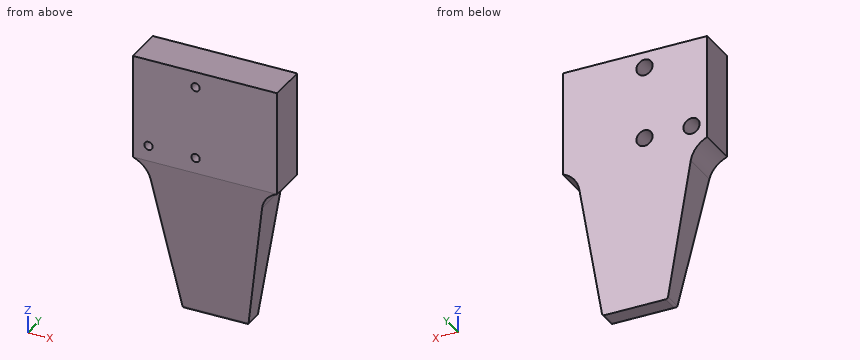
from build123d import *

# Parameters (mm, degrees)
SKETCH1_W           = 55.25
SKETCH1_H           = 100
SKETCH1_R           = 1.6
BOSS_EXTRUDE1_DEPTH = 15
SKETCH2_R           = 3.1
CUT_EXTRUDE1_DEPTH  = 7.5
CUT_EXTRUDE3_REACH  = 117.228
CUT_EXTRUDE2_REACH  = 117.228
FILLET3_R           = 10
FILLET4_R           = 1


with BuildPart() as part:
    # Sketch1 → Boss-Extrude1 (new body)
    with BuildSketch(Plane(origin=(0, 0, 0), x_dir=(1, 0, 0), z_dir=(0, 1, 0))):
        with Locations((27.625, 50)):
            Rectangle(SKETCH1_W, SKETCH1_H)
        with Locations(Location((24, 6, 0), (0, 0, 270))):
            Circle(SKETCH1_R, mode=Mode.SUBTRACT)
        with Locations(Location((6, 34, 0), (0, 0, 270))):
            Circle(SKETCH1_R, mode=Mode.SUBTRACT)
        with Locations(Location((24, 34, 0), (0, 0, 270))):
            Circle(SKETCH1_R, mode=Mode.SUBTRACT)
    extrude(amount=BOSS_EXTRUDE1_DEPTH)

    # Sketch2 → Cut-Extrude1 (cut)
    with BuildSketch(Plane(origin=(0, 15, 0), x_dir=(1, 0, 0), z_dir=(0, 1, 0))):
        with Locations(Location((24, 34, 0), (0, 0, 270))):
            Circle(SKETCH2_R)
        with Locations(Location((24, 6, 0), (0, 0, 270))):
            Circle(SKETCH2_R)
        with Locations(Location((6, 34, 0), (0, 0, 270))):
            Circle(SKETCH2_R)
    extrude(amount=-CUT_EXTRUDE1_DEPTH, mode=Mode.SUBTRACT)

    # Sketch5 → Cut-Extrude3 (cut, up to next)
    with BuildSketch(Plane(origin=(55.25, 0, 0), x_dir=(0, 0, -1), z_dir=(1, 0, 0)), mode=Mode.PRIVATE) as cut_extrude3_sk1:
        Polygon((40, 0), (100, 8), (100, 0), align=None)
    cut_extrude3_tool1 = extrude(cut_extrude3_sk1.sketch, amount=-CUT_EXTRUDE3_REACH, mode=Mode.PRIVATE) & part.part
    add(cut_extrude3_tool1.solids().sort_by_distance((55.25, 2.666667, -80))[0], mode=Mode.SUBTRACT)

    # Sketch3 → Cut-Extrude2 (cut, up to next)
    with BuildSketch(Plane(origin=(0, 15, 0), x_dir=(1, 0, 0), z_dir=(0, 1, 0)), mode=Mode.PRIVATE) as cut_extrude2_sk1:
        Polygon((40.125, 100), (55.25, 100), (55.25, 40), (50.25, 40), align=None)
    cut_extrude2_tool1 = extrude(cut_extrude2_sk1.sketch, amount=-CUT_EXTRUDE2_REACH, mode=Mode.PRIVATE) & part.part
    # Sketch3 → Cut-Extrude2 (cut, up to next)
    with BuildSketch(Plane(origin=(0, 15, 0), x_dir=(1, 0, 0), z_dir=(0, 1, 0)), mode=Mode.PRIVATE) as cut_extrude2_sk2:
        Polygon((15.125, 100), (0, 100), (0, 40), (5, 40), align=None)
    cut_extrude2_tool2 = extrude(cut_extrude2_sk2.sketch, amount=-CUT_EXTRUDE2_REACH, mode=Mode.PRIVATE) & part.part
    add(cut_extrude2_tool1.solids().sort_by_distance((49.794255, 15, -75.031056))[0], mode=Mode.SUBTRACT)
    add(cut_extrude2_tool2.solids().sort_by_distance((5.455745, 15, -75.031056))[0], mode=Mode.SUBTRACT)

    # Fillet3
    # the kernel refuses this fillet: 10 mm, written as the material it adds along each edge
    with BuildSketch(Plane(origin=(5, 15, -40), x_dir=(-1, 0, 0), z_dir=(0, -1, 0))) as fillet3_piece_1_section:
        with BuildLine():
            CenterArc((8.564743476, 9.343051105), FILLET3_R, 189.578422919, 59.537746257)
            Line((-1.295844232, 7.679076929), (-1.493055986, 7.645797446))
            Line((-1.493055986, 7.645797446), (-0.197211754, -0.033279484))
            Line((-0.197211754, -0.033279484), (0, -0.2))
            ThreePointArc((0, -0.2), (2.5, -0.2), (4.92870513, -0.186861022))
            Line((4.92870513, -0.186861022), (5, 0))
        make_face()
    fillet3_piece_1 = extrude(amount=15, mode=Mode.PRIVATE)
    fillet3_piece_1 = split(fillet3_piece_1, bisect_by=Plane(origin=(4.040002964, 0.373004519, -42.797533893), z_dir=(0, 0.9912279006826347, 0.13216372009101796)), keep=Keep.TOP, mode=Mode.PRIVATE)
    add(fillet3_piece_1)
    with BuildSketch(Plane(origin=(50.25, 15, -40), x_dir=(1, 0, 0), z_dir=(0, -1, 0))) as fillet3_piece_2_section:
        with BuildLine():
            CenterArc((8.564743476, -9.343051105), FILLET3_R, 110.883830823, 59.537746257)
            Line((-1.295844232, -7.679076929), (-1.493055986, -7.645797446))
            Line((-1.493055986, -7.645797446), (-0.197211754, 0.033279484))
            Line((-0.197211754, 0.033279484), (0, 0.2))
            ThreePointArc((0, 0.2), (2.5, 0.2), (4.92870513, 0.186861022))
            Line((4.92870513, 0.186861022), (5, 0))
        make_face()
    fillet3_piece_2 = extrude(amount=15, mode=Mode.PRIVATE)
    fillet3_piece_2 = split(fillet3_piece_2, bisect_by=Plane(origin=(51.209997036, 0.373004519, -42.797533893), z_dir=(0, 0.9912279006826347, 0.13216372009101796)), keep=Keep.TOP, mode=Mode.PRIVATE)
    add(fillet3_piece_2)

    # Fillet4
    fillet4_edges = [part.edges().sort_by_distance(p)[0] for p in [
        (27.625, 8, -100),
        (15.125, 11.5, -100),
        (40.125, 11.5, -100),
    ]]
    fillet(fillet4_edges, radius=FILLET4_R)


solid = part.part
Geometry: final body of the model. Coordinates: model frame, mm. Round coordinates to 2 decimals unless told otherwise and drop trailing zeros. Loops run counter-clockwise (first coordinate to the right, second up) from the corner with the lowest first, then second, coordinate; pieces in that order, holes last. Notation, with made-up numbers: M 55.25,12.5 L 64.25,12.5 A22 cw 64.25,25.5 Z; hole C 39,82 d3. An arc over 180 degrees is marked long. One line per question, with ' | ' between items.
(1) Cut plane A-A on z = -6. Return the cut outline in (x, y), plus the area to 3 significant figures.
Check result:
outline: M 0,0 L 22.4,0 L 22.4,7.5 L 20.9,7.5 L 20.9,15 L 0,15 Z; M 25.6,0 L 55.25,0 L 55.25,15 L 27.1,15 L 27.1,7.5 L 25.6,7.5 Z | area: 758 mm2
(2) Contact query for flat-ended pins moving along their axis: P1, Ø3.5, axis at x = 24, z = -34, coming from the +Y side; P2, Ø6, axis at x = 18, y = 5.5, coming from the -Z side; P3, Ø8, axis at y = 8, z = -49.5, coming from the +X side. Output: stop coordinate, or through.
Check result:
P1: stops at y = 7.5 | P2: stops at z = -99.93 | P3: stops at x = 49.58
(3) Cut plane D-D on z = -34. Return the cut outline in (x, y).
Check result:
outline: M 0,0 L 4.4,0 L 4.4,7.5 L 2.9,7.5 L 2.9,15 L 0,15 Z; M 7.6,0 L 22.4,0 L 22.4,7.5 L 20.9,7.5 L 20.9,15 L 9.1,15 L 9.1,7.5 L 7.6,7.5 Z; M 25.6,0 L 55.25,0 L 55.25,15 L 27.1,15 L 27.1,7.5 L 25.6,7.5 Z
(4) Cut plane B-B on x = 24. Return the cut outline in (y, z).
Check result:
outline: M 0,-40 L 7.88,-99.13 A1 ccw 8.88,-100 L 15,-100 L 15,-37.1 L 7.5,-37.1 L 7.5,-35.6 L 0,-35.6 Z; M 0,-32.4 L 7.5,-32.4 L 7.5,-30.9 L 15,-30.9 L 15,-9.1 L 7.5,-9.1 L 7.5,-7.6 L 0,-7.6 Z; M 0,-4.4 L 7.5,-4.4 L 7.5,-2.9 L 15,-2.9 L 15,0 L 0,0 Z
(5) Material intervals for line 1 along X through (y, z) = (12, -34); line 2 along X through (y, z) = (4, -34); line 3 along X through (y, z) = (4, -6), sorted ascending. Write a range as from..to.
Check result:
line 1: x = 0..2.9, 9.1..20.9, 27.1..55.25 | line 2: x = 0..4.4, 7.6..22.4, 25.6..55.25 | line 3: x = 0..22.4, 25.6..55.25
(6) Cut plane C-C on y = 13.5. Return the cut outline in (x, z), plus the area to 3 significant figures.
Check result:
outline: M 0,-40 A10 cw 6.3,-47.68 L 14.98,-99.17 A1 ccw 15.97,-100 L 39.28,-100 A1 ccw 40.27,-99.17 L 48.95,-47.68 A10 cw 55.25,-40 L 55.25,0 L 0,0 Z; hole C 6,-34 d6.2; hole C 24,-34 d6.2; hole C 24,-6 d6.2 | area: 4,250 mm2
